Source: CAD feature listing. Evaluate the final solid. Frame: model axes, mm. Give positions to 0.01 mm unless a question says otherwise; leave off trailing zeros. Write each loop counter-clockwise with the first axis right and the second up, starting at its lowest first coordinate (ties: lowest second). Pieces come first, ordered by that corner, then holes. Notation, with made-up numbers: (77.25, 37) -> (86.25, 37) arc R20 cw to (86.25, 55) -> close; hole circle Ø11 at (-32.5, 69.5). An arc over 180 degrees is marked (long way). Answer as a JSON object with one key per item and string values. Group by question number.
Item 1: Section query C-C on y = 26.4. Return the cut outline in (x, z), plus the area to 3 significant figures.
Item 2: Section query B-B on x = 27.25. Return the cut outline in (y, z).
Item 3: Section query D-D on z = 0.55. Return the cut outline in (x, y).
Item 4: Ray query, probe 1 along Y at (x, z) = (25.93, 0.5); probe 2 along X at (y, z) = (26.4, 0.3); probe 3 along Y at (x, z) = (27.25, 0.3). Return the intervals inside material, ascending. Write a range as from..to.
Item 5: Section query A-A on y = 23. Return the cut outline in (x, z).
Autodesk Inventor part; units mm, degrees
ref_plane "BoardFrontPlane" through (0, 0, 0) normal (0, 0, 1) x (1, 0, 0)
ref_plane "YZ Plane" through (0, 0, 0) normal (1, 0, 0) x (0, 1, 0)
ref_plane "XZ Plane" through (0, 0, 0) normal (0, 1, 0) x (-1, 0, 0)
ref_plane "BoardFrontPlane" through (0, 0, 0) normal (0, 0, 1) x (1, 0, 0)
sketch "Sketch1" plane through (0, 0, 0) normal (0, 0, 1) x (1, 0, 0)
  line L0 (24, 22.5) -> (24, 42.5)
  arc A0 (25.5, 44) -> (24, 42.5) centre (25.5, 42.5) ccw
  line L1 (25.5, 44) -> (29, 44)
  arc A1 (30.5, 42.5) -> (29, 44) centre (29, 42.5) ccw
  line L2 (30.5, 42.5) -> (30.5, 22.5)
  arc A2 (29, 21) -> (30.5, 22.5) centre (29, 22.5) ccw
  line L3 (29, 21) -> (25.5, 21)
  arc A3 (24, 22.5) -> (25.5, 21) centre (25.5, 22.5) ccw
extrude "BoardOutline" add sketch "Sketch1" along normal blind 0.798
sketch "img_Top" plane through (0, 0, 0.798) normal (0, 0, 1) x (1, 0, 0)
  line L0 (24, 44) -> (30.4988, 44) construction
  line L1 (30.4988, 44) -> (30.4988, 21) construction
  line L2 (30.4988, 21) -> (24, 21) construction
  line L3 (24, 21) -> (24, 44) construction
decal "Decal_Top"
sketch "img_Bottom" plane through (0, 0, -0.798) normal (0, 0, -1) x (1, 0, 0)
  line L0 (24, -21) -> (30.4988, -21) construction
  line L1 (30.4988, -21) -> (30.4988, -44) construction
  line L2 (30.4988, -44) -> (24, -44) construction
  line L3 (24, -44) -> (24, -21) construction
decal "Decal_Bottom"
sketch "Sketch4" plane through (0, 0, 0.798) normal (0, 0, 1) x (1, 0, 0)
  point P0 (28.47, 26.4)
hole "Q1-2" at (28.47, 26.4, 0.798) direction (0, 0, -1) diameter 0.9652 end through all
sketch "Sketch5" plane through (0, 0, 0.798) normal (0, 0, 1) x (1, 0, 0)
  point P0 (25.93, 26.4)
hole "Q1-1" at (25.93, 26.4, 0.798) direction (0, 0, -1) diameter 0.9652 end through all
sketch "Sketch6" plane through (0, 0, 0.798) normal (0, 0, 1) x (1, 0, 0)
  point P0 (28.47, 38.6)
hole "LED1-1" at (28.47, 38.6, 0.798) direction (0, 0, -1) diameter 0.9652 end through all
sketch "Sketch7" plane through (0, 0, 0.798) normal (0, 0, 1) x (1, 0, 0)
  point P0 (25.93, 38.6)
hole "LED1-2" at (25.93, 38.6, 0.798) direction (0, 0, -1) diameter 0.9652 end through all
sketch "Sketch8" plane through (0, 0, 0.798) normal (0, 0, 1) x (1, 0, 0)
  point P0 (27.25, 42)
hole "Free-MP2" at (27.25, 42, 0.798) direction (0, 0, -1) diameter 2.2 end through all
sketch "Sketch9" plane through (0, 0, 0.798) normal (0, 0, 1) x (1, 0, 0)
  point P0 (27.25, 23)
hole "Free-MP1" at (27.25, 23, 0.798) direction (0, 0, -1) diameter 2.2 end through all
properties part number "ND.ForageFeeder.BeamBreak_BOARD"
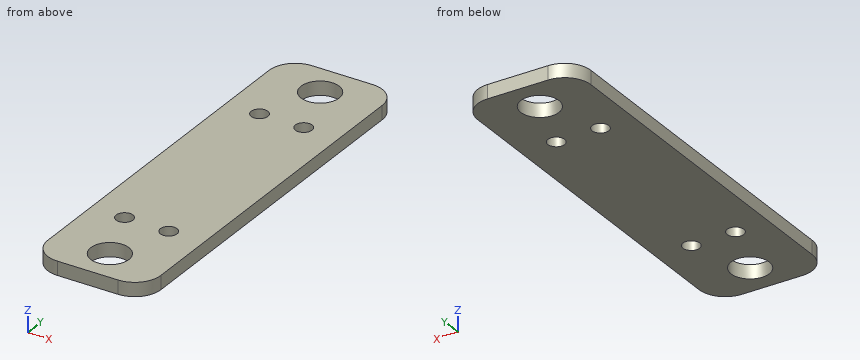
Worked answers:
{
 "1": {"outline": "(24, 0) -> (25.45, 0) -> (25.45, 0.8) -> (24, 0.8) -> close; (26.41, 0) -> (27.99, 0) -> (27.99, 0.8) -> (26.41, 0.8) -> close; (28.95, 0) -> (30.5, 0) -> (30.5, 0.8) -> (28.95, 0.8) -> close", "area": "3.65 mm^2"},
 "2": {"outline": "(21, 0) -> (21.9, 0) -> (21.9, 0.8) -> (21, 0.8) -> close; (24.1, 0) -> (40.9, 0) -> (40.9, 0.8) -> (24.1, 0.8) -> close; (43.1, 0) -> (44, 0) -> (44, 0.8) -> (43.1, 0.8) -> close"},
 "3": {"outline": "(24, 22.5) arc R1.5 ccw to (25.5, 21) -> (29, 21) arc R1.5 ccw to (30.5, 22.5) -> (30.5, 42.5) arc R1.5 ccw to (29, 44) -> (25.5, 44) arc R1.5 ccw to (24, 42.5) -> close; hole circle Ø0.97 at (25.93, 26.4); hole circle Ø0.97 at (25.93, 38.6); hole circle Ø2.2 at (27.25, 23); hole circle Ø2.2 at (27.25, 42); hole circle Ø0.97 at (28.47, 26.4); hole circle Ø0.97 at (28.47, 38.6)"},
 "4": {"probe 1": "21..25.92, 26.88..38.12, 39.08..44", "probe 2": "24..25.45, 26.41..27.99, 28.95..30.5", "probe 3": "21..21.9, 24.1..40.9, 43.1..44"},
 "5": {"outline": "(24, 0) -> (26.15, 0) -> (26.15, 0.8) -> (24, 0.8) -> close; (28.35, 0) -> (30.5, 0) -> (30.5, 0.8) -> (28.35, 0.8) -> close"}
}
